Geometry check sheet. Reference: the model listing, model coordinates, mm. Round coordinates to 2 decimals unless told otherwise and drop trailing zeros. Order: outer loops, then holes, each group sorted by start corner. A loop starts at its lowest first (then second) coordinate and runs counter-clockwise, first axis right, second up. Notation, with made-up numbers: (72, 27.25) -> (89, 27.25) arc R7 cw to (89, 31.25) -> close; hole circle Ø3 at (-39.75, 70.5). An arc over 180 degrees is marked (long way). Answer as a JSON object with one key per item and string values. Group by question number.
from build123d import *

# Parameters (mm, degrees)
EXTRUDE_1_DEPTH          = 300
EXTRUDE_1_DEPTH_BACK     = 300
SKETCH_1_R               = 4
SKETCH_1_R_2             = 3
CUT_EXTRUDE_2_DEPTH      = 301.053328593
CUT_EXTRUDE_2_DEPTH_BACK = 301.053328593
SKETCH_3_R               = 1


with BuildPart() as part:
    # Sketch 1 → Extrude 1 (new, two sides: drawn at the far end of the back side and taken through both)
    with BuildSketch(Plane.XY.offset(-EXTRUDE_1_DEPTH_BACK)):
        Circle(SKETCH_1_R)
        Circle(SKETCH_1_R_2, mode=Mode.SUBTRACT)
    extrude(amount=EXTRUDE_1_DEPTH + EXTRUDE_1_DEPTH_BACK)

    # Sketch 3 → Cut-Extrude 2 (cut, two sides: drawn at the far end of the back side and taken through both)
    with BuildSketch(Plane(origin=(0, 0, 0), x_dir=(1, 0, 0), z_dir=(0, 1, 0)).offset(-CUT_EXTRUDE_2_DEPTH_BACK)):
        with Locations(Location((0, 295, 0), (0, 0, 270))):
            Circle(SKETCH_3_R)
        with Locations(Location((0, -295, 0), (0, 0, 270))):
            Circle(SKETCH_3_R)
    extrude(amount=CUT_EXTRUDE_2_DEPTH + CUT_EXTRUDE_2_DEPTH_BACK, mode=Mode.SUBTRACT)


solid = part.part
Item 1: Sectioned sample at B-B, the plane z = -83. Enter the section's corners in (x, y).
Item 2: Sectioned sample at A-A, the plane y = 0. Enter the section's corners in (x, z), then the cut area to 3 significant figures.
Item 3: Depth check by flat-ended pin: pin 1 Ø2 at (y, z) = (2, 30) entering from -X; pin 2 Ø3 at (x, z) = (-2, -7) entering from +Y; pin 3 Ø2 at (y, z) = (-3, 146) entering from -X. Enter the tip coordinate at first touch or a pass-through.
Item 4: Thickness scan on L1, parallel to Z at x = 0, y = -3.5; L2, parallel to Y at x = 0.25, z = -153; L3, parallel to X at y = -0.75, z = -119.5. Record the ranges inside material, lowest first.
Result:
{
 "1": {"outline": "circle Ø8 at (0, 0); hole circle Ø6 at (0, 0)"},
 "2": {"outline": "(-4, -300) -> (-3, -300) -> (-3, 300) -> (-4, 300) -> close; (3, -300) -> (4, -300) -> (4, 300) -> (3, 300) -> close", "area": "1,200 mm2"},
 "3": {"pin 1": "stops at x = -3.87", "pin 2": "stops at y = 3.97", "pin 3": "stops at x = -3.46"},
 "4": {"L1": "z = -300 to -296, -294 to 294, 296 to 300", "L2": "y = -3.99 to -2.99, 2.99 to 3.99", "L3": "x = -3.93 to -2.9, 2.9 to 3.93"}
}
